The listing builds one solid part. Answer for the finished solid, in the listing's coordinates (mm). Round coordinates to 2 decimals unless told otherwise and drop trailing zeros. Write each loop counter-clockwise with the first axis right and the second up, starting at its lowest first coordinate (ties: lowest second). Pieces come first, ordered by that corner, then holes. Notation, with made-up numbers: (-29, 4.5) - (24, 4.5) arc R5 ccw to (24, 12.5) - close; hole circle Ø10 at (-23, 28). An arc over 180 degrees is marked (long way). Answer in a Markdown table with one row per item.
from build123d import *

# Parameters (mm, degrees)
F0_R     = 10
F2_DEPTH = 1000
F1_R     = 9
F3_DEPTH = 1000.001
F4_DEPTH = 1000.001


with BuildPart() as f2:
    # F0 (on Top) → F2 (new body, symmetric)
    with BuildSketch(Plane.XY):
        Circle(F0_R)
    extrude(amount=F2_DEPTH, both=True)

    # F1 (on Top) → F3 (cut, through all)
    with BuildSketch(Plane.XY):
        Circle(F1_R)
    extrude(amount=-F3_DEPTH, mode=Mode.SUBTRACT)

    # F1 (on Top) → F4 (cut, through all)
    with BuildSketch(Plane.XY):
        Circle(F1_R)
    extrude(amount=F4_DEPTH, mode=Mode.SUBTRACT)


solid = f2.part
(1) Flat-ended cylindrical pins translate along their axes: pin 1 (4 mm diameter, centred on x = 8, z = 426.5, fed in from +Y); pin 2 (4 mm diameter, centred on x = 5.5, z = -232.5, fed in from +Y); pin 3 (3 mm diameter, centred on x = 5, z = -309.5, fed in from -Y). Find the tip coordinate at first contact, or state that the pin passes through.
Checked values:
| item | result |
|---|---|
| pin 1 | stops at y = 8 |
| pin 2 | stops at y = 9.37 |
| pin 3 | stops at y = -9.37 |
(2) Section C-C (z = 340.5) is taken. Give the vertices of the cut face in (x, y), and give its area (3 significant figures).
Checked values:
| item | result |
|---|---|
| outline | circle Ø20 at (0, 0); hole circle Ø18 at (0, 0) |
| area | 59.7 mm2 |
(3) Section A-A (x = 0) is taken. Give the vertices of the cut face in (y, z), and give its area (3 significant figures).
Checked values:
| item | result |
|---|---|
| outline | (-10, -1000) - (-9, -1000) - (-9, 1000) - (-10, 1000) - close; (9, -1000) - (10, -1000) - (10, 1000) - (9, 1000) - close |
| area | 4,000 mm2 |
(4) Find the intervals of material crossed by line 1 (Y direction, x = 0, z = -318); line 2 (X direction, y = 1, z = 76); line 3 (Y direction, x = -2.5, z = -397.5), in increasing order.
Checked values:
| item | result |
|---|---|
| line 1 | y = -10 to -9, 9 to 10 |
| line 2 | x = -9.95 to -8.94, 8.94 to 9.95 |
| line 3 | y = -9.68 to -8.65, 8.65 to 9.68 |
